The model under review builds one solid part; all positions refer to its coordinate system, in mm. A direction names the side the tool comes from. Round coordinates to 2 decimals unless told otherwise and drop trailing zeros. Write each loop counter-clockwise with the first axis right and the second up, starting at its lowest first coordinate (ties: lowest second). Pieces come first, ordered by that corner, then holes. Notation, with made-up numbers: (55, 44) -> (96, 44) arc R38 ccw to (96, 83) -> close; hole circle Ø5 at (57, 82.25). An arc over 180 degrees is marked (long way). Return JSON: item names as keys, results as strings. Group by question number.
1. Mouldability with a two-part tool opening along X and no side actions: class faces 1 (the cylindrical face through (0.66, 1.486, -14.985)), 2 (the cylindrical face through (0.526, 2.746, -8.331)), 3 (the cylindrical face through (-4.88, 12.34, -1.08)), 4 (the flat face through (2, 25, -5)) as pulls with the +X half, pulls with the -X half, needs draft (parallel to the pull), parting line crosses it, or undercut.
2. For line 1 along X through (y, z) = (17.25, 0); line 2 along Y through (x, z) = (9, -5.5); line 3 along Z through (x, y) = (-4, 5), list the stretches that pass through material, from the lowest coordinate up. Write a range as from..to.
3. Tool access review of faces 5 (the cylindrical face through (0.526, 2.746, 8.331)), 6 (the flat face through (-3, 3, -7)): name each direction out of +Z, -Z, +X, -X, +Y, -Y from which nothing blocks a thin tool from reaching the whole face with its end or side.
4. Take a section at A-A, the plane z = 0. Write out the cut boundary in (x, y), then the cut area to 3 significant figures.
5. Clearance check with flat-ended pins moving along their axes: P1, Ø4, axis at x = 0, z = -10, coming from the +Y side; P2, Ø1.5, axis at y = 12, z = -4.5, coming from the +X side; P3, Ø1, axis at y = 4.5, z = -6.5, coming from the +X side. State where each tip first meets the part, or that it passes through.
6. Take a section at B-B, the plane y = 14.5. Write out the cut boundary in (x, z).
from build123d import *

# Parameters (mm, degrees)
SKETCH_1_R                   = 15
SKETCH_1_R_2                 = 5
EXTRUDE_1_DEPTH              = 3
SKETCH_1_3_R                 = 7
SKETCH_1_3_R_2               = 5
EXTRUDE_2_DEPTH              = 25
SKETCH_2_R                   = 1.75
CUT_EXTRUDE_1_DEPTH          = 33.787192622
CHAMFER_1_SIZE               = 2.5
CHAMFER_1_OF_MIRROR_659_SIZE = 2.5
CHAMFER_2_SIZE               = 2
CHAMFER_2_SIZE2              = 0.535898385
CHAMFER_4_SIZE               = 1
CHAMFER_4_SIZE2              = 0.176326981
CHAMFER_5_SIZE               = 0.5


with BuildPart() as part:
    # Sketch 1 → Extrude 1 (new body)
    with BuildSketch(Plane(origin=(0, 0, 0), x_dir=(1, 0, 0), z_dir=(0, 1, 0))):
        with Locations(Location((0, 0, 0), (0, 0, 270))):
            Circle(SKETCH_1_R)
        with Locations(Location((0, 0, 0), (0, 0, 270))):
            Circle(SKETCH_1_R_2, mode=Mode.SUBTRACT)
    extrude(amount=EXTRUDE_1_DEPTH)

    # Sketch 1_3 → Extrude 2 (add)
    with BuildSketch(Plane(origin=(0, 0, 0), x_dir=(1, 0, 0), z_dir=(0, 1, 0))):
        with Locations(Location((0, 0, 0), (0, 0, 270))):
            Circle(SKETCH_1_3_R)
        with Locations(Location((0, 0, 0), (0, 0, 270))):
            Circle(SKETCH_1_3_R_2, mode=Mode.SUBTRACT)
    extrude(amount=EXTRUDE_2_DEPTH)

    # Sketch 2 → Cut-Extrude 1 (cut, through all)
    with BuildSketch(Plane.XZ):
        with Locations(Location((0, 10, 0), (0, 0, 270))):
            Circle(SKETCH_2_R)
    cut_extrude_1 = extrude(amount=-CUT_EXTRUDE_1_DEPTH, mode=Mode.SUBTRACT)

    # Chamfer 1
    chamfer_1_edges = [part.edges().sort_by_distance(p)[0] for p in [
        (0, 0, 11.75),
    ]]
    chamfer(chamfer_1_edges, length=CHAMFER_1_SIZE)

    # Mirror 659: Cut-Extrude 1 across plane
    add(cut_extrude_1.mirror(Plane.XY), mode=Mode.SUBTRACT)

    # Chamfer 1 of Mirror 659
    chamfer_1_of_mirror_659_edges = [part.edges().sort_by_distance(p)[0] for p in [
        (0, 0, -11.75),
    ]]
    chamfer(chamfer_1_of_mirror_659_edges, length=CHAMFER_1_OF_MIRROR_659_SIZE)

    # Chamfer 2
    chamfer_2_edges = [part.edges().sort_by_distance(p)[0] for p in [
        (0, 25, -7),
    ]]
    chamfer_2_side = [part.faces().sort_by_distance(p)[0] for p in [
        (0, 14, -7),
    ]]
    chamfer(chamfer_2_edges, length=CHAMFER_2_SIZE, length2=CHAMFER_2_SIZE2, reference=chamfer_2_side[0])

    # Chamfer 4
    chamfer_4_edges = [part.edges().sort_by_distance(p)[0] for p in [
        (0, 25, -5),
        (0, 0, -5),
    ]]
    chamfer_4_side = [part.faces().sort_by_distance(p)[0] for p in [
        (0, 12.5, -5),
    ]]
    chamfer(chamfer_4_edges, length=CHAMFER_4_SIZE, length2=CHAMFER_4_SIZE2, reference=chamfer_4_side[0])

    # Chamfer 5
    chamfer_5_edges = [part.edges().sort_by_distance(p)[0] for p in [
        (0, 0, -15),
        (0, 3, -15),
    ]]
    chamfer(chamfer_5_edges, length=CHAMFER_5_SIZE)


solid = part.part
Output:
{
 "1": {"face 1": "parting line crosses it", "face 2": "undercut", "face 3": "undercut", "face 4": "needs draft"},
 "2": {"line 1": "x = -7..-5, 5..7", "line 2": "y = 0..3", "line 3": "z = -5.74..-3, 3..5.74"},
 "3": {"face 5": "+Y, -Y", "face 6": "+Y"},
 "4": {"outline": "(-15, 0.5) -> (-14.5, 0) -> (-5.18, 0) -> (-5, 1) -> (-5, 24) -> (-5.18, 25) -> (-6.46, 25) -> (-7, 23) -> (-7, 3) -> (-14.5, 3) -> (-15, 2.5) -> close; (5, 1) -> (5.18, 0) -> (14.5, 0) -> (15, 0.5) -> (15, 2.5) -> (14.5, 3) -> (7, 3) -> (7, 23) -> (6.46, 25) -> (5.18, 25) -> (5, 24) -> close", "area": "146 mm^2"},
 "5": {"P1": "stops at y = 3", "P2": "stops at x = 5.91", "P3": "stops at x = 3.61"},
 "6": {"outline": "circle Ø14 at (0, 0); hole circle Ø10 at (0, 0)"}
}
